Build history of the part. All positions in model axes, mm. A direction names the side the tool comes from. Round coordinates to 2 decimals unless told otherwise and drop trailing zeros. Order: outer loops, then holes, each group sorted by start corner. A loop starts at its lowest first (then second) coordinate and runs counter-clockwise, first axis right, second up. Notation, with made-up numbers: (-34.75, -24.75) -> (-10.75, -24.75) arc R13 cw to (-10.75, -15.75) -> close; hole circle Ø4 at (-18, 17.5). An arc over 180 degrees is marked (long way). Write item = value, one per line.
from build123d import *

# Parameters (mm, degrees)
SKETCH1_R             = 13.5
BOSS_EXTRUDE1_DEPTH   = 3
F_2_0MM_DOWEL_HOLE1_D = 2


with BuildPart() as part:
    # Sketch1 → Boss-Extrude1 (new body)
    with BuildSketch(Plane.XY):
        with BuildLine():
            Line((-20, 123.389626793), (-20, 6.305975778))
            Line((-20, 6.305975778), (-87.156423304, -89.603336304))
            ThreePointArc((-87.156423304, -89.603336304), (-37.588224938, -119.214618844), (20, -123.389626793))
            Line((20, -123.389626793), (20, -77.459666924))
            ThreePointArc((20, -77.459666924), (76.29735606, -24.05646396), (60.812080601, 51.979715784))
            Line((60.812080601, 51.979715784), (87.156423304, 89.603336304))
            ThreePointArc((87.156423304, 89.603336304), (37.588224938, 119.214618844), (-20, 123.389626793))
        make_face()
        with Locations((0, -97.082039325)):
            Circle(SKETCH1_R, mode=Mode.SUBTRACT)
        with Locations((43.59255168, -37.082039325)):
            Circle(SKETCH1_R, mode=Mode.SUBTRACT)
        with BuildLine():
            ThreePointArc((32.5, 0), (30.995800899, -9.772938484), (26.622441439, -18.641234181))
            ThreePointArc((26.622441439, -18.641234181), (23.140620238, -19.255173201), (22.526681218, -15.773352))
            ThreePointArc((22.526681218, -15.773352), (26.227216146, -8.269409486), (27.5, 0))
            ThreePointArc((27.5, 0), (30, 2.5), (32.5, 0))
        make_face(mode=Mode.SUBTRACT)
        with Locations((43.59255168, 37.082039325)):
            Circle(SKETCH1_R, mode=Mode.SUBTRACT)
        with Locations((0, 97.082039325)):
            Circle(SKETCH1_R, mode=Mode.SUBTRACT)
    extrude(amount=BOSS_EXTRUDE1_DEPTH)

    # Ø2.0mm Dowel Hole1 (through all)
    with Locations(Plane.XY.offset(3)):
        with Locations((0, -10), (10, 0), (0, 10), (0, 0), (-10, 0)):
            Hole(F_2_0MM_DOWEL_HOLE1_D / 2)


solid = part.part
Q1. Cut at C-C, the plane y = -81. List the corners of the cut face in (x, z), and give its area (3 significant figures).
Check values:
outline = (-81.13, 0) -> (20, 0) -> (20, 3) -> (-81.13, 3) -> close
area = 303 mm²
Q2. Cut at B-B, the plane z = 1.65. Give the number of separate pieces and of enclosed holes in the cut face, and give its area (3 significant figures).
Check values:
separate_pieces = 1
enclosed_holes = 10
area = 21,900 mm²
Q3. Flat gauge pins, fed straight in: pin 1 (1 mm diameter, centred on y = -60, z = 2.5, fed in from -X); pin 2 (0.9 mm diameter, centred on y = -95.5, z = 1, fed in from +X); pin 3 (1 mm diameter, centred on y = 64.5, z = 0.5, fed in from +X). Where does each tip first touch, or does it go through?
Check values:
pin_1 = -66.78
pin_2 = 20
pin_3 = 69.93
Q4. Cut at A-A, the plane x = 36. List the corners of the cut face in (y, z), and give its area (3 significant figures).
Check values:
outline = (-71.44, 0) -> (-48.24, 0) -> (-48.24, 3) -> (-71.44, 3) -> close; (-25.92, 0) -> (25.92, 0) -> (25.92, 3) -> (-25.92, 3) -> close; (48.24, 0) -> (119.7, 0) -> (119.7, 3) -> (48.24, 3) -> close
area = 439 mm²
Q5. Which spindle directions (+Z, -Z, +X, -X, +Y, -Y) get a long thin tool onto all of the face, cutting with end or side? Do faces 1 (the face through (26.19, -8.38, 1.48)), 2 (the face through (-1, 2, 0)). Say none if no direction does.
Check values:
face_1 = +Z, -Z
face_2 = -Z, +X, -X, +Y, -Y
Q6. Mould opens along X. For faces 3 (the face through (73.8, 70.53, 1.48)), 4 (the face through (-1, 2, 3)), 5 (the face through (31.037, -9.64, 1.479)), 6 (the face through (-38.365, -118.967, 1.479)) say: released by +X, released by -X, zero draft, split by the parting line, or undercut.
Check values:
face_3 = released by +X
face_4 = zero draft
face_5 = undercut
face_6 = split by the parting line
Q7. Cut at D-D, the plane x = -76. List the corners of the cut face in (y, z).
Check values:
outline = (-99.24, 0) -> (-73.67, 0) -> (-73.67, 3) -> (-99.24, 3) -> close
Q8. Probe probe 1 along Y at (x, z) = (0, 1.7); probe 2 along Y at (x, z) = (-12, 1.2); probe 3 along Y at (x, z) = (-1.5, 0.35). List the from-to ranges inside material, lowest first.
Check values:
probe_1 = -125 to -110.58, -83.58 to -11, -9 to -1, 1 to 9, 11 to 83.58, 110.58 to 125
probe_2 = -124.42 to -103.27, -90.9 to 90.9, 103.27 to 124.42
probe_3 = -124.99 to -110.5, -83.67 to 83.67, 110.5 to 124.99
